Here's how the part is built. I have some questions about the finished solid (model axes, mm). Face numbers are marked on the shaded views. A direction names the side the tool comes from. Round coordinates to 2 decimals unless told otherwise and drop trailing zeros. Loops run counter-clockwise (first coordinate to the right, second up) from the corner with the lowest first, then second, coordinate; pieces in that order, holes last. Notation, with made-up numbers: M 85,30 L 110,30 A8 cw 110,40 Z; hole C -1.5,40.5 d10. An arc over 180 degrees is marked long. Answer as a JSON object with one key per item and string values.
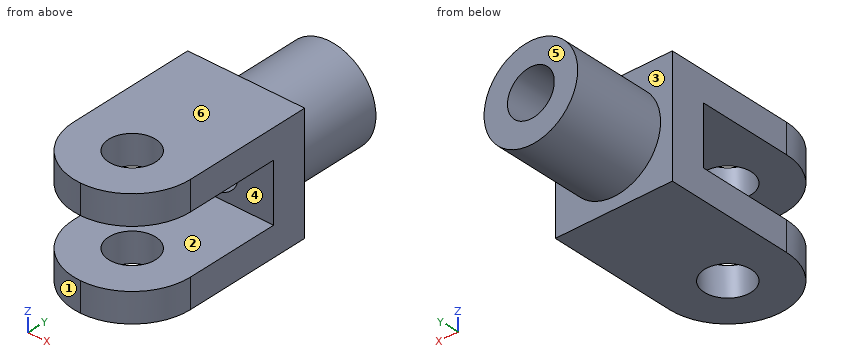
from build123d import *

# Parameters (mm, degrees)
F0_W     = 50
F0_H     = 50
F1_DEPTH = 7.5
F2_W     = 50
F2_H     = 12.5
F3_DEPTH = 65
F5_D     = 20
F6_R     = 25
F7_R     = 24.99999
F8_R     = 20
F9_DEPTH = 40
F11_D    = 20


# Not quite as in the source:
# - a fillet or chamfer is up to 0.001 mm smaller than in the source, because OpenCascade refuses the exact size


with BuildPart() as f1:
    # F0 (on Front) → F1 (new body, symmetric)
    with BuildSketch(Plane.XZ):
        Rectangle(F0_W, F0_H)
    extrude(amount=F1_DEPTH, both=True)

    # F2 (on face) → F3 (join)
    with BuildSketch(Plane.XZ.offset(7.5)):
        with Locations((0, -18.75)):
            Rectangle(F2_W, F2_H)
        with Locations((0, 18.75)):
            Rectangle(F2_W, F2_H)
    extrude(amount=F3_DEPTH)

    # F5 (through all)
    with Locations(Plane.XY.offset(25)):
        with Locations((0, -47.5)):
            Hole(F5_D / 2)

    # F6
    f6_edges = [f1.edges().sort_by_distance(p)[0] for p in [
        (-25, -72.5, -18.75),
    ]]
    fillet(f6_edges, radius=F6_R)

    # F7 (radius 25 in the source; OpenCascade refuses exactly that, so slightly less here)
    f7_edges = [f1.edges().sort_by_distance(p)[0] for p in [
        (25, -72.5, 18.75),
        (25, -72.5, -18.75),
        (-25, -72.5, 18.75),
    ]]
    fillet(f7_edges, radius=F7_R)

    # F8 (on face) → F9 (join)
    with BuildSketch(Plane(origin=(0, 7.5, 0), x_dir=(-1, 0, 0), z_dir=(0, 1, 0))):
        Circle(F8_R)
    extrude(amount=F9_DEPTH)

    # F11 (through all)
    with Locations(Plane(origin=(0, 47.5, 0), x_dir=(-1, 0, 0), z_dir=(0, 1, 0))):
        with Locations((0, 0)):
            Hole(F11_D / 2)


solid = f1.part
Item 1: On a 3-axis mill with a long thin cutter (end or side, diameter ignored), from which of +Z, -Z, +X, -X, +Y, -Y can I reach the whole of each face in a straight line? I mean the marked faces 1, 2 and 3. Say none if no direction works.
Resolved:
{"face 1": "+Z, -Z, -X, -Y", "face 2": "+X, -X, -Y", "face 3": "+Y"}
Item 2: If we mould it in two halves opening along Z, with no side actions, what happens to the marked faces 4, 5 and 6? For each: pulls with the +Z half, pulls with the -Z half, needs draft (parallel to the pull), parting line crosses it, or undercut.
Resolved:
{"face 4": "undercut", "face 5": "needs draft", "face 6": "pulls with the +Z half"}
Item 3: I want a section at D-D, the plane y = -60. Please give me the cut outline in (x, z), then the cut area to 3 significant figures.
Resolved:
{"outline": "M -21.65,-25 L 21.65,-25 L 21.65,-12.5 L -21.65,-12.5 Z; M -21.65,12.5 L 21.65,12.5 L 21.65,25 L -21.65,25 Z", "area": "1,080 mm²"}
Item 4: Please list where these lines run through material, in increasing order: probe 1 along Z at (x, y) = (5.5, -66.5); probe 2 along Z at (x, y) = (0, 24); probe 3 along Y at (x, z) = (-10, -7). Write a range as from..to.
Resolved:
{"probe 1": "-25..-12.5, 12.5..25", "probe 2": "-20..-10, 10..20", "probe 3": "-7.5..47.5"}
Item 5: I'm going to push flat-ended pins straight in: pin 1 Ø8 at (x, z) = (16.5, 14.5) entering from -Y; pin 2 Ø4 at (x, y) = (-12, 14.5) entering from +Z; pin 3 Ø20 at (x, z) = (8, 0.5) entering from -Y. Where does each tip first touch, or does it pass through?
Resolved:
{"pin 1": "y = -69.15", "pin 2": "z = 17.32", "pin 3": "y = -7.5"}
Item 6: I want a section at B-B, the plane y = 0. Please give me the cut outline in (x, z).
Resolved:
{"outline": "M -25,-25 L 25,-25 L 25,25 L -25,25 Z; hole C 0,0 d20"}
Item 7: I want a section at C-C, the plane x = 7. Please give me the cut outline in (y, z) (3 decimals).
Resolved:
{"outline": "M -71.5,-25 L -54.641,-25 L -54.641,-12.5 L -71.5,-12.5 Z; M -71.5,12.5 L -54.641,12.5 L -54.641,25 L -71.5,25 Z; M -40.359,-25 L 7.5,-25 L 7.5,-18.735 L 47.5,-18.735 L 47.5,-7.141 L -7.5,-7.141 L -7.5,-12.5 L -40.359,-12.5 Z; M -40.359,12.5 L -7.5,12.5 L -7.5,7.141 L 47.5,7.141 L 47.5,18.735 L 7.5,18.735 L 7.5,25 L -40.359,25 Z"}
Item 8: I want a section at A-A, the plane z = 0. Please give me the cut outline in (x, y).
Resolved:
{"outline": "M -25,-7.5 L -10,-7.5 L -10,47.5 L -20,47.5 L -20,7.5 L -25,7.5 Z; M 10,-7.5 L 25,-7.5 L 25,7.5 L 20,7.5 L 20,47.5 L 10,47.5 Z"}
